```python
from build123d import *

# Parameters (mm, degrees)
BOSS_EXTRUDE1_DEPTH = 20.32


with BuildPart() as part:
    # Sketch1 → Boss-Extrude1 (new body)
    with BuildSketch(Plane(origin=(0, 0, 0), x_dir=(1, 0, 0), z_dir=(0, 1, 0))):
        with BuildLine():
            Line((-72.961668905, 52.840505094), (-222.399785176, 133.135612345))
            ThreePointArc((-222.399785176, 133.135612345), (-270.024680251, 147.912216254), (-231.416447367, 116.354602156))
            Line((-231.416447367, 116.354602156), (-81.978331095, 36.059494906))
            ThreePointArc((-81.978331095, 36.059494906), (-60.41841965, 0), (-81.978331095, -36.059494906))
            Line((-81.978331095, -36.059494906), (-231.416447367, -116.354602156))
            ThreePointArc((-231.416447367, -116.354602156), (-270.024680251, -147.912216254), (-222.399785176, -133.135612345))
            Line((-222.399785176, -133.135612345), (-72.961668905, -52.840505094))
            Line((-72.961668905, -52.840505094), (-55.765211733, -52.840505094))
            Line((-55.765211733, -52.840505094), (-38.625312425, -127.499494906))
            Line((-38.625312425, -127.499494906), (0, -127.499494906))
            Line((0, -127.499494906), (38.625312425, -127.499494906))
            Line((38.625312425, -127.499494906), (55.765211733, -52.840505094))
            Line((55.765211733, -52.840505094), (72.961668905, -52.840505094))
            Line((72.961668905, -52.840505094), (222.399785176, -133.135612345))
            ThreePointArc((222.399785176, -133.135612345), (270.024680251, -147.912216254), (231.416447367, -116.354602156))
            Line((231.416447367, -116.354602156), (81.978331095, -36.059494906))
            ThreePointArc((81.978331095, -36.059494906), (60.41841965, 0), (81.978331095, 36.059494906))
            Line((81.978331095, 36.059494906), (231.416447367, 116.354602156))
            ThreePointArc((231.416447367, 116.354602156), (270.024680251, 147.912216254), (222.399785176, 133.135612345))
            Line((222.399785176, 133.135612345), (72.961668905, 52.840505094))
            Line((72.961668905, 52.840505094), (31.75, 141.740505094))
            Line((31.75, 141.740505094), (-31.75, 141.740505094))
            Line((-31.75, 141.740505094), (-72.961668905, 52.840505094))
        make_face()
    extrude(amount=BOSS_EXTRUDE1_DEPTH)


solid = part.part
```
Build history of the part. All positions in model axes, mm. A direction names the side the tool comes from. Coordinates: 2 decimals unless noted, no trailing zeros. Order: outer loops, then holes, each group sorted by start corner. A loop starts at its lowest first (then second) coordinate and runs counter-clockwise, first axis right, second up. Notation, with made-up numbers: (4.25, -13) -> (25.25, -13) arc R16 ccw to (25.25, -2) -> close; hole circle Ø1 at (-33.5, -15). An arc over 180 degrees is marked (long way). Answer in a Markdown table with one row per item. Add a question column.
Q1. Band-saw the part on D-D, the plane x = -236.5. List the corners of the cut face in (y, z).
Q2. Band-saw the part on A-A, the plane x = 247.65. List the corners of the cut face in (y, z), then the cut area to 3 significant figures.
Q3. Drop flat-ended pins along their axis: pin 1 (6 mm diameter, centred on y = 6.5, z = 122.5, fed in from +X); pin 2 (10 mm diameter, centred on y = 5.5, z = -40, fed in from +X); pin 3 (8.5 mm diameter, centred on x = -61.5, y = 6.5, fed in from +Z). Give the stop position or say it passes through.
Q4. Mould opens along X. For faces 4 (the face through (-60.423, 10.018, -0.618)), 5 (the face through (0, 10, -141.741)), 6 (the face through (-1, 0, -1)) say: +X half, -X half, draft (parallel to the pull), parting line (faces both ways), or undercut.
Q5. Wall check: line 1 along X through (y, z) = (7.75, -120); line 2 along X through (y, z) = (18.75, -59); line 3 along Z through (x, y) = (157, 12). Give the ranges that are in metal, low to high. Write a range as [from, to].
Q6. Which spindle directions (+Z, -Z, +X, -X, +Y, -Y) get a long thin tool onto all of the face, cutting with end or side? Do faces 1 (the face through (-52.07, 10.02, -97.91)), 2 (the face through (-64, 10, 52.841)), 3 (the face through (-1, 20.32, -1)). Say none if no direction does.
Q7. Band-saw the part on C-C, the plane y = 6.75. List the corners of the cut face in (x, z).
Q8. Band-saw the part on B-B, the plane z = -58. List the corners of the cut face in (x, y).
Answers follow:
| question | item | result |
|---|---|---|
| 1 | outline | (0, -158.71) -> (20.32, -158.71) -> (20.32, -113.07) -> (0, -113.07) -> close; (0, 113.07) -> (20.32, 113.07) -> (20.32, 158.71) -> (0, 158.71) -> close |
| 2 | outline | (0, -161.29) -> (20.32, -161.29) -> (20.32, -110.49) -> (0, -110.49) -> close; (0, 110.49) -> (20.32, 110.49) -> (20.32, 161.29) -> (0, 161.29) -> close |
| 2 | area | 2,060 mm^2 |
| 3 | pin 1 | x = 270.83 |
| 3 | pin 2 | x = 98.62 |
| 3 | pin 3 | z = 52.84 |
| 4 | face 4 | -X half |
| 4 | face 5 | undercut |
| 4 | face 6 | draft |
| 5 | line 1 | [-267.47, -197.95], [-41.83, 41.83], [197.95, 267.47] |
| 5 | line 2 | [-124.67, -84.43], [-70.11, 70.11], [84.43, 124.67] |
| 5 | line 3 | [-98, -76.37], [76.37, 98] |
| 6 | face 1 | -Z, +Y, -Y |
| 6 | face 2 | +Z, +Y, -Y |
| 6 | face 3 | +Z, -Z, +X, -X, +Y |
| 7 | outline | (-231.42, -116.35) arc R25.4 ccw (long way) to (-222.4, -133.14) -> (-72.96, -52.84) -> (-31.75, -141.74) -> (31.75, -141.74) -> (72.96, -52.84) -> (222.4, -133.14) arc R25.4 ccw (long way) to (231.42, -116.35) -> (81.98, -36.06) arc R40.94 cw to (81.98, 36.06) -> (231.42, 116.35) arc R25.4 ccw (long way) to (222.4, 133.14) -> (72.96, 52.84) -> (55.77, 52.84) -> (38.63, 127.5) -> (-38.63, 127.5) -> (-55.77, 52.84) -> (-72.96, 52.84) -> (-222.4, 133.14) arc R25.4 ccw (long way) to (-231.42, 116.35) -> (-81.98, 36.06) arc R40.94 cw to (-81.98, -36.06) -> close |
| 8 | outline | (-122.81, 0) -> (-82.56, 0) -> (-82.56, 20.32) -> (-122.81, 20.32) -> close; (-70.57, 0) -> (70.57, 0) -> (70.57, 20.32) -> (-70.57, 20.32) -> close; (82.56, 0) -> (122.81, 0) -> (122.81, 20.32) -> (82.56, 20.32) -> close |
